Design review of the part built by this model. Coordinates are the model's own, in mm. A direction names the side the tool comes from. Coordinates: 2 decimals unless noted, no trailing zeros. Write each loop counter-clockwise with the first axis right and the second up, starting at its lowest first coordinate (ties: lowest second). Pieces come first, ordered by that corner, then holes.
Q1. Take a section at A-A (x = 28). Give the boundary of the cut face in (y, z).
Q2. Take a section at D-D (x = 16). Give the boundary of the cut face in (y, z), and give its area (3 significant figures).
Q3. Take a section at C-C (z = 21.5). Give the boundary of the cut face in (x, y), and give its area (3 significant figures).
Q4. Insertion check: pin 1 (3 mm diameter, centred on x = 4.5, z = 6, fed in from -Y); pin 2 (1.5 mm diameter, centred on x = 9.5, z = -7.5, fed in from +Y); pin 3 (6 mm diameter, centred on x = 26, z = 8, fed in from +Y); pin 4 (5.5 mm diameter, centred on y = 0, z = 15, fed in from -X) (3 decimals). Each pin has a flat end and moves straight along its axis. Give the tip position at first contact, or say it passes through.
Q5. For probe 1 along Y at (x, z) = (16, -3); probe 2 along X at (y, z) = (3.75, 19); probe 3 along Z at (x, y) = (30.65, 0), list the stretches that pass through material, from the lowest coordinate up.
Q6. Take a section at B-B (y = -0.75). Give the boundary of the cut face in (x, z).
Q7. Mouldability with a two-part tool opening along X and no side actions: class faces 1 (the flat face through (16, -1, 0)), 2 (the flat face through (16, 8, 4)), 3 (the flat face through (32, 0, 11)) as pulls with the +X half, pulls with the -X half, needs draft (parallel to the pull), parting line crosses it, or undercut.
Q8. Machinability: for faces 4 (the flat face through (16.1, -8.4, 0)), 5 (the flat face through (5, -2, 12)), 6 (the cylindrical face through (7.416, 2.703, -5.423)), which of the approach directions +Z, -Z, +X, -X, +Y, -Y give a long, thin tool a straight path to every point of the face, cutting with its end or side? Answer none if there is none.
```python
from build123d import *

# Parameters (mm, degrees)
F0_W     = 9
F0_H     = 11
F2_DEPTH = 8
F4_DEPTH = 11
F5_R     = 3
F6_DEPTH = 32.001


# Not quite as in the source:
# - a feature names something its author has since deleted; it is built from what else it names


with BuildPart() as f1:
    # F0 (on Front) → F1 (revolve)
    with BuildSketch(Plane.XZ):
        with Locations((11.5, -5.5)):
            Rectangle(F0_W, F0_H)
    revolve(axis=Axis((16, 0, -5.5), (0, 0, -1)))

    # F0 (on Front) → F2 (join, symmetric)
    with BuildSketch(Plane.XZ):
        Polygon((0, 23), (0, 0), (7, 0), (16, 0), (32, 0), (32, 23), (27, 23), (27, 6), (5, 6), (5, 23), align=None)
    extrude(amount=F2_DEPTH, both=True)

    # F3 (on face) → F4 (cut)
    with BuildSketch(Plane(origin=(0, 0, -11), x_dir=(1, 0, 0), z_dir=(0, 0, -1))):
        with BuildLine():
            Line((14.5, 6.2696960071), (14.5, 4.7696960071))
            ThreePointArc((14.5, 4.7696960071), (16, -5), (17.5, 4.7696960071))
            Line((17.5, 4.7696960071), (17.5, 6.2696960071))
            Line((17.5, 6.2696960071), (14.5, 6.2696960071))
        make_face()
    extrude(amount=-F4_DEPTH, mode=Mode.SUBTRACT)

    # F5 (on face) → F6 (cut, through all)
    with BuildSketch(Plane.YZ.offset(32)):
        with Locations((0, 15)):
            Circle(F5_R)
        with BuildLine():
            ThreePointArc((-8, 15), (-5.6568542495, 20.6568542495), (0, 23))
            Line((0, 23), (-8, 23))
            Line((-8, 23), (-8, 15))
        make_face()
        with BuildLine():
            ThreePointArc((0, 23), (5.6568542495, 20.6568542495), (8, 15))
            Line((8, 15), (8, 23))
            Line((8, 23), (0, 23))
        make_face()
    extrude(amount=-F6_DEPTH, mode=Mode.SUBTRACT)


solid = f1.part
```
Response:
1. outline: (-8, 0) - (8, 0) - (8, 15) arc R8 ccw to (-8, 15) - close; hole circle Ø6 at (0, 15)
2. outline: (-9, -11) - (-6.27, -11) - (-6.27, 0) - (5, 0) - (5, -11) - (9, -11) - (9, 0) - (8, 0) - (8, 6) - (-8, 6) - (-8, 0) - (-9, 0) - close
2. area: 170 mm2
3. outline: (0, -4.66) - (5, -4.66) - (5, 4.66) - (0, 4.66) - close; (27, -4.66) - (32, -4.66) - (32, 4.66) - (27, 4.66) - close
3. area: 93.3 mm2
4. pin 1: stops at y = -8
4. pin 2: stops at y = 6.92
4. pin 3: stops at y = 8
4. pin 4: passes through
5. probe 1: y = -9 to -6.27, 5 to 9
5. probe 2: x = 0 to 5, 27 to 32
5. probe 3: z = 0 to 12, 18 to 23
6. outline: (0, 0) - (7.03, 0) - (7.03, -11) - (11.06, -11) - (11.06, 0) - (20.94, 0) - (20.94, -11) - (24.97, -11) - (24.97, 0) - (32, 0) - (32, 12.1) - (27, 12.1) - (27, 6) - (5, 6) - (5, 12.1) - (0, 12.1) - close; (0, 17.9) - (5, 17.9) - (5, 22.96) - (0, 22.96) - close; (27, 17.9) - (32, 17.9) - (32, 22.96) - (27, 22.96) - close
7. face 1: undercut
7. face 2: needs draft
7. face 3: pulls with the +X half
8. face 4: +Z, +X, -X, -Y
8. face 5: +Z, +Y, -Y
8. face 6: -Z
